Could you check a few things on this model? Use its own coordinates, in mm. A direction names the side the tool comes from. Give positions to 0.01 mm unless a question says otherwise; leave off trailing zeros. Write each loop counter-clockwise with the first axis right and the second up, starting at its lowest first coordinate (ties: lowest second). Pieces come first, ordered by that corner, then holes. Notation, with made-up numbers: M 20.5,63 L 36.5,63 A26 cw 36.5,91 Z; hole C 30.5,80.5 d11. An arc over 180 degrees is marked long. Use one line per item in the form item = value.
from build123d import *

# Parameters (mm, degrees)
BOSS_EXTRUDE3_DEPTH  = 4
BOSS_EXTRUDE30_DEPTH = 2.1
CUT_EXTRUDE23_DEPTH  = 19.67655379
CUT_EXTRUDE24_DEPTH  = 18.444111581


with BuildPart() as part:
    # Sketch3<4> → Boss-Extrude3 (new body)
    with BuildSketch(Plane(origin=(0, 0.5, 0), x_dir=(1, 0, 0), z_dir=(0, 1, 0))):
        Polygon((5.617596648, 2.37486125), (5.073087868, 7.275440269), (2.993112649, 9.355415488), (1.620820393, 12.1), (-1.620820393, 12.1), (-2.993112649, 9.355415488), (-5.073087868, 7.275440269), (-5.617596648, 2.37486125), (-3.951674234, -0.6), (3.951674234, -0.6), align=None)
        Polygon((-4.5, 7), (-5, 2.5), (-3.599999905, 0), (3.599999905, 0), (5, 2.5), (4.5, 7), (2.5, 9), (1.25, 11.5), (-1.25, 11.5), (-2.5, 9), align=None, mode=Mode.SUBTRACT)
    extrude(amount=-BOSS_EXTRUDE3_DEPTH)

    # Sketch57 → Boss-Extrude30 (add)
    with BuildSketch(Plane(origin=(0, 0.5, 0), x_dir=(1, 0, 0), z_dir=(0, 1, 0))):
        Polygon((-8.022942498, 6.351803212), (-8.022942498, 1.811803212), (-5.075187344, -2.1), (5.075187344, -2.1), (8.022942498, 1.811803212), (8.022942498, 6.351803212), (5.075187344, 10.263606425), (-5.075187344, 10.263606425), align=None)
    extrude(amount=BOSS_EXTRUDE30_DEPTH)

    # Sweep3: sweep along a path in Sketch3
    with BuildLine(Plane(origin=(0, 0.5, 0), x_dir=(1, 0, 0), z_dir=(0, 1, 0))) as sweep3_path:
        Line((-4.5, 7), (-5, 2.5))
        Line((-5, 2.5), (-3.599999905, 0))
        Line((-3.599999905, 0), (3.599999905, 0))
        Line((3.599999905, 0), (5, 2.5))
        Line((5, 2.5), (4.5, 7))
        Line((4.5, 7), (2.5, 9))
        Line((2.5, 9), (1.25, 11.5))
        Line((1.25, 11.5), (-1.25, 11.5))
        Line((-1.25, 11.5), (-2.5, 9))
        Line((-2.5, 9), (-4.5, 7))
    # Sketch4 → Sweep3 (sweep)
    with BuildSketch(Plane(origin=(0, 0, 0), x_dir=(0, 0, -1), z_dir=(1, 0, 0))):
        Polygon((0, 0.5), (-0.6, 0.5), (-2.62762332, 2.52762332), (-4.32762332, 2.52762332), (-4.32762332, 3.12762332), (-2.62762332, 3.12762332), align=None)
    sweep(path=sweep3_path.line, transition=Transition.RIGHT)

    # Cut-Sweep10: sweep along a path in Sketch61
    with BuildLine(Plane(origin=(0, 0.5, 0), x_dir=(1, 0, 0), z_dir=(0, 1, 0))) as cut_sweep10_path:
        Line((1.25, 11.5), (2.5, 9))
        Line((2.5, 9), (4.5, 7))
        Line((4.5, 7), (5, 2.5))
        Line((5, 2.5), (3.599999905, 0))
        Line((3.599999905, 0), (-3.599999905, 0))
        Line((-3.599999905, 0), (-5, 2.5))
        Line((-5, 2.5), (-4.5, 7))
        Line((-4.5, 7), (-2.5, 9))
        Line((-2.5, 9), (-1.25, 11.5))
        Line((-1.25, 11.5), (1.25, 11.5))
    # Sketch60 → Cut-Sweep10 (sweep, cut)
    with BuildSketch(Plane(origin=(0, 0, 0), x_dir=(0, 0, -1), z_dir=(1, 0, 0))):
        Polygon((-4.32762332, 3.12762332), (-2.62762332, 3.12762332), (0, 0.5), (0.419943975, 0.080056025), (0.419943975, 3.72762332), (0, 3.72762332), (-4.32762332, 3.72762332), align=None)
    sweep(path=cut_sweep10_path.line, transition=Transition.RIGHT, mode=Mode.SUBTRACT)


with BuildPart() as cut_sweep10_kept_piece:
    # of the separate pieces the step leaves, the one the design keeps (cut_sweep10_pieces_kept)
    add(part.part.solids().sort_by_distance((5.617596648, 0.5, -2.37486125))[0])

    # Sketch62 → Cut-Extrude23 (cut, symmetric)
    with BuildSketch(Plane(origin=(0.147112643, 0, -0.195225071), x_dir=(0, -1, 0), z_dir=(0.6018150231520525, 0, -0.7986355100472898))):
        Polygon((-2.52762332, 10.230017371), (-2.52762332, 11.230017371), (-0.5, 11.230017371), (-0.5, 10.230017371), (-0.96381166, 9.766205711), (-2.06381166, 9.766205711), align=None)
    extrude(amount=CUT_EXTRUDE23_DEPTH, both=True, mode=Mode.SUBTRACT)

    # Sketch64 → Cut-Extrude24 (cut, symmetric)
    with BuildSketch(Plane(origin=(-3.776568435, 0, -5.011675586), x_dir=(0, -1, 0), z_dir=(-0.6018150231520465, 0, -0.7986355100472943))):
        Polygon((-2.52762332, 5.317036382), (-2.52762332, 6.317036382), (-0.5, 6.317036382), (-0.5, 5.317036382), (-0.96381166, 4.853224722), (-2.06381166, 4.853224722), align=None)
    extrude(amount=CUT_EXTRUDE24_DEPTH, both=True, mode=Mode.SUBTRACT)


solid = cut_sweep10_kept_piece.part
1) If I drill on L1, parallel to Z at x = 1, y = -0.75; L2, parallel to X at y = 1.25, z = -6.75; L3, parallel to X at y = -0.75, z = -8, over which ranges is the centre line in solid material (lowest first)?
Checked values:
L1 = -12.1 to -11.5, 0 to 0.6
L2 = -7.14 to -5.28, 5.28 to 7.72
L3 = -4.35 to -3.5, 3.5 to 4.35
2) I want a section at C-C, the plane x = -1. Please give me the cut outline in (y, z), plus the area to 3 significant figures.
Checked values:
outline = M -3.5,-12.1 L 0.5,-12.1 L 2.53,-14.13 L 2.53,-15.83 L 3.13,-15.83 L 3.13,-14.13 L 0.5,-11.5 L -3.5,-11.5 Z; M -3.5,0 L 0.5,0 L 3.13,2.63 L 3.13,4.33 L 2.53,4.33 L 2.53,2.63 L 2,2.1 L 0.5,2.1 L 0.5,0.6 L -3.5,0.6 Z
area = 10.8 mm2
3) Thinking about a two-plate mould opening in Z: for faces 5 (the flat face through (5.5, 2.4, 1.72)), 6 (the flat face through (-6.417, 2.292, -8.093)), 7 (the flat face through (0.1, 1.8, 1.3)), which applies, released by +Z, released by -Z, zero draft, split by the parting line, or undercut?
Checked values:
face_5 = released by +Z
face_6 = released by -Z
face_7 = undercut
4) I want a section at B-B, the plane z = -1. Please give me the cut outline in (x, y).
Checked values:
outline = M -9.12,2.53 L -7.41,2.53 L -6.83,2.06 L -6.83,0.96 L -7.41,0.5 L -4.85,0.5 L -4.85,-3.5 L -4.16,-3.5 L -4.16,0.5 L -7.17,3.13 L -9.12,3.13 Z; M 4.16,-3.5 L 4.85,-3.5 L 4.85,0.5 L 7.41,0.5 L 7.41,2.53 L 9.12,2.53 L 9.12,3.13 L 7.17,3.13 L 4.16,0.5 Z
5) For pin 1 Ø6 at (x, z) = (-0.5, -4) entering from -Y; pin 2 Ø1.2 at (x, y) = (-0.5, -2) entering from +Z; pin 3 Ø2.5 at (x, y) = (0, -1.5) entering from -Z; pin 4 Ø2 at (y, z) = (2, -4) entering from +X, each with a flat end and sliding along its axis, tell me the tip position at first contact or that it passes through.
Checked values:
pin_1 = through
pin_2 = 0.6
pin_3 = -12.1
pin_4 = 9.28
6) I want a section at A-A, the plane y = 0.25. Please give me the cut outline in (x, z), plus the area to 3 significant figures.
Checked values:
outline = M -5.62,-2.37 L -5.07,-7.28 L -2.99,-9.36 L -1.62,-12.1 L 1.62,-12.1 L 2.99,-9.36 L 5.07,-7.28 L 5.62,-2.37 L 3.95,0.6 L -3.95,0.6 Z; hole M -5,-2.5 L -4.5,-7 L -2.5,-9 L -1.25,-11.5 L 1.25,-11.5 L 2.5,-9 L 4.5,-7 L 5,-2.5 L 3.6,0 L -3.6,0 Z
area = 22.7 mm2
7) For faces 1 (the flat face through (-2.297, -1.472, -10.747)), 2 (the flat face through (2, -1, -10)), 3 (the flat face through (-8.023, 1, -4)), 4 (the flat face through (-6.37, 2.29, -0.01)), which set-ups out of +Z, -Z, +X, -X, +Y, -Y let a thin tool reach every point of the face, with its end or its side?
Checked values:
face_1 = -Z, -X, -Y
face_2 = +Y, -Y
face_3 = +Z, -Z, -X, -Y
face_4 = +Z, -X
8) I want a section at D-D, the plane z = -3.5. Please give me the cut outline in (x, y).
Checked values:
outline = M -9.24,2.53 L -8.02,2.53 L -8.02,0.5 L -5.49,0.5 L -5.49,-3.5 L -4.89,-3.5 L -4.89,0.5 L -7.53,3.13 L -9.24,3.13 Z; M 4.89,-3.5 L 5.49,-3.5 L 5.49,0.5 L 8.02,0.5 L 8.02,2.53 L 9.24,2.53 L 9.24,3.13 L 7.53,3.13 L 4.89,0.5 Z
